Part model, mm, in its own coordinate system. A direction names the side the tool comes from. Round coordinates to 2 decimals unless told otherwise and drop trailing zeros. Write each loop counter-clockwise with the first axis right and the second up, starting at its lowest first coordinate (ties: lowest second). Pieces come first, ordered by that corner, then holes.
1) Saw through at C-C on z = -0.5. Write the cut outline in (x, y), and give its area (3 significant figures).
2) Drill centre lines: L1, parallel to X at y = 18.5, z = 2.25; L2, parallel to Y at x = 10.75, z = 7.35; L3, parallel to Z at x = -2.5, y = 13.5. Where is each one in solid material? Low to high.
3) Flat gauge pins, fed straight in: pin 1 (3 mm diameter, centred on y = 23.5, z = 6, fed in from +X); pin 2 (1.5 mm diameter, centred on x = 11.5, y = 22.5, fed in from -Z); pin 3 (4 mm diameter, centred on y = 24.5, z = 4, fed in from -X); pin 4 (8 mm diameter, centred on x = 11.5, y = 13, fed in from +Z). Where does each tip first touch, or does it go through?
4) Saw through at D-D on x = 10.5. Write the cut outline in (y, z).
5) Which spindle directions (+Z, -Z, +X, -X, +Y, -Y) get a long thin tool onto all of the face, cutting with end or side? Do faces 4 (the flat face through (0, 27, 7)), 5 (the flat face through (6.25, 19, 2)), 6 (the flat face through (-6.25, 19, 2)), 7 (the flat face through (0, 17, 5.5)). Say none if no direction does.
6) Pull direction Y, two halves, no side cores. Call faces 1 (the cylindrical face through (-4.729, 22.233, -0.24)), 2 (the flat face through (-11, 17, 5.5)), 3 (the cylindrical face through (12.969, 24.594, 6.979)): +Y half, -Y half, draft (parallel to the pull), parting line (faces both ways), or undercut.
7) Saw through at B-B on y = 13. Write the cut outline in (x, z), and give its area (3 significant figures).
8) Saw through at A-A on z = 5. Write the cut outline in (x, y).
```python
from build123d import *

# Parameters (mm, degrees)
EXTRUDE_1_DEPTH     = 27
SKETCH_3_R          = 2
CUT_EXTRUDE_2_DEPTH = 31.943496894
FILLET_1_R          = 5
SKETCH_4_W          = 9
SKETCH_4_H          = 27
SKETCH_4_R          = 1.5
EXTRUDE_2_DEPTH     = 3
FILLET_2_R          = 8
SKETCH_5_W          = 38.66542969
SKETCH_5_H          = 14
CUT_EXTRUDE_3_DEPTH = 36.363293116
FILLET_3_R          = 5
FILLET_4_R          = 8
SKETCH_6_R          = 12.5
CUT_EXTRUDE_5_DEPTH = 36.545745174
FILLET_5_R          = 5


with BuildPart() as part:
    # 草图1 → 凸台-拉伸1 (new body)
    with BuildSketch(Plane(origin=(0, 0, 0), x_dir=(1, 0, 0), z_dir=(0, 1, 0))):
        Polygon((-6.25, 8.5), (-6.25, -8.5), (6.25, -8.5), (6.25, 8.5), (3.25, 8.5), (3.25, -5.5), (-3.25, -5.5), (-3.25, 8.5), align=None)
    extrude(amount=EXTRUDE_1_DEPTH)

    # 草图3 → 切除-拉伸2 (cut, through all)
    with BuildSketch(Plane(origin=(6.25, 0, 0), x_dir=(0, 0, -1), z_dir=(1, 0, 0))):
        with Locations((0.5, 20.25)):
            Circle(SKETCH_3_R)
    extrude(amount=-CUT_EXTRUDE_2_DEPTH, mode=Mode.SUBTRACT)

    # 圆角1
    fillet_1_edges = [part.edges().sort_by_distance(p)[0] for p in [
        (-4.75, 0, -8.5),
        (4.75, 0, -8.5),
        (-4.75, 27, -8.5),
        (4.75, 27, -8.5),
    ]]
    fillet(fillet_1_edges, radius=FILLET_1_R)

    # 草图4 → 凸台-拉伸2 (add)
    # profile 1 of 2: a face of its own
    with BuildSketch(Plane.XY.offset(8.5)):
        with Locations((-10.75, 13.5)):
            Rectangle(SKETCH_4_W, SKETCH_4_H)
        with Locations((-10.75, 13)):
            Circle(SKETCH_4_R, mode=Mode.SUBTRACT)
        with Locations((-10.75, 21)):
            Circle(SKETCH_4_R, mode=Mode.SUBTRACT)
    # profile 2 of 2: a face of its own
    with BuildSketch(Plane.XY.offset(8.5)):
        with Locations((10.75, 13.5)):
            Rectangle(SKETCH_4_W, SKETCH_4_H)
        with Locations((10.75, 13)):
            Circle(SKETCH_4_R, mode=Mode.SUBTRACT)
        with Locations((10.75, 21)):
            Circle(SKETCH_4_R, mode=Mode.SUBTRACT)
    extrude(amount=-EXTRUDE_2_DEPTH)

    # 圆角2
    fillet_2_edges = [part.edges().sort_by_distance(p)[0] for p in [
        (-15.25, 27, 7),
        (15.25, 27, 7),
    ]]
    fillet(fillet_2_edges, radius=FILLET_2_R)

    # 草图5 → 切除-拉伸3 (cut, through all)
    with BuildSketch(Plane.XY.offset(8.5)):
        Rectangle(SKETCH_5_W, SKETCH_5_H)
    extrude(amount=-CUT_EXTRUDE_3_DEPTH, mode=Mode.SUBTRACT)

    # 圆角3
    fillet_3_edges = [part.edges().sort_by_distance(p)[0] for p in [
        (4.75, 7, -8.5),
        (-4.75, 7, -8.5),
    ]]
    fillet(fillet_3_edges, radius=FILLET_3_R)

    # 圆角4
    fillet_4_edges = [part.edges().sort_by_distance(p)[0] for p in [
        (-15.25, 7, 7),
        (15.25, 7, 7),
    ]]
    fillet(fillet_4_edges, radius=FILLET_4_R)

    # 草图6 → 切除-拉伸5 (cut, through all)
    with BuildSketch(Plane(origin=(6.25, 0, 0), x_dir=(0, 0, -1), z_dir=(1, 0, 0))):
        with Locations((8.5, 5)):
            Circle(SKETCH_6_R)
    extrude(amount=-CUT_EXTRUDE_5_DEPTH, mode=Mode.SUBTRACT)

    # 圆角5
    fillet_5_edges = [part.edges().sort_by_distance(p)[0] for p in [
        (4.75, 17.5, -8.5),
        (-4.75, 17.5, -8.5),
    ]]
    fillet(fillet_5_edges, radius=FILLET_5_R)


solid = part.part
```
Completed:
1. outline: (-6.25, 14.6) - (-3.25, 14.6) - (-3.25, 18.25) - (-6.25, 18.25) - close; (-6.25, 22.25) - (-3.25, 22.25) - (-3.25, 27) - (-6.25, 27) - close; (3.25, 14.6) - (6.25, 14.6) - (6.25, 18.25) - (3.25, 18.25) - close; (3.25, 22.25) - (6.25, 22.25) - (6.25, 27) - (3.25, 27) - close
1. area: 50.4 mm2
2. L1: x = -6.25 to -3.25, 3.25 to 6.25
2. L2: y = 7.81 to 11.5, 14.5 to 19.5, 22.5 to 26.19
2. L3: z = 5.5 to 8.5
3. pin 1: stops at x = 14.67
3. pin 2: stops at z = 5.5
3. pin 3: stops at x = -14.07
3. pin 4: stops at z = 8.5
4. outline: (7.69, 5.5) - (11.52, 5.5) - (11.52, 8.5) - (7.69, 8.5) - close; (14.48, 5.5) - (19.52, 5.5) - (19.52, 8.5) - (14.48, 8.5) - close; (22.48, 5.5) - (26.31, 5.5) - (26.31, 8.5) - (22.48, 8.5) - close
5. face 4: +Z, -Z, +X, -X, +Y
5. face 5: -Z, +X, +Y, -Y
5. face 6: -Z, -X, +Y, -Y
5. face 7: -Z, +Y, -Y
6. face 1: undercut
6. face 2: draft
6. face 3: +Y half
7. outline: (-15, 5.5) - (-12.25, 5.5) - (-12.25, 8.5) - (-15, 8.5) - close; (-9.25, 5.5) - (-6.25, 5.5) - (-6.25, 1.1) - (-3.25, 1.1) - (-3.25, 5.5) - (3.25, 5.5) - (3.25, 1.1) - (6.25, 1.1) - (6.25, 5.5) - (9.25, 5.5) - (9.25, 8.5) - (-9.25, 8.5) - close; (12.25, 5.5) - (15, 5.5) - (15, 8.5) - (12.25, 8.5) - close
7. area: 98.3 mm2
8. outline: (-6.25, 7) - (-3.25, 7) - (-3.25, 27) - (-6.25, 27) - close; (3.25, 7) - (6.25, 7) - (6.25, 27) - (3.25, 27) - close
